For this review, take the finished solid that the model builds, in its own axes (mm). Face numbers are marked on the shaded views. A direction names the side the tool comes from. Coordinates: 2 decimals unless noted, no trailing zeros. Loops run counter-clockwise (first coordinate to the right, second up) from the corner with the lowest first, then second, coordinate; pieces in that order, holes last. Notation, with made-up numbers: (43, 47) - (62, 47) arc R20 cw to (62, 56) - close; hole circle Ø11 at (-23, 20). An arc over 180 degrees is marked (long way). One line per item, written item: value. Start each with the question number.
1. Take a section at A-A, the plane x = 4. State the section outline as (y, z) points, and give its area (3 significant figures).
2. The part is to be moulded in two halves that separate along X. For the marked faces 6, 7 and 8, say which applies: released by +X, released by -X, zero draft, split by the parting line, or undercut.
3. To check wall thickness, follow line 1 (Y direction, x = -3, z = 1.5); line 2 (Y direction, x = 1, z = 4.5); line 3 (X direction, y = -13.5, z = 3). State the ranges of each line that lie inside material, in increasing order. Write a range as from..to.
4. Insertion check: pin 1 (1.5 mm diameter, centred on y = -3, z = 1, fed in from -X); pin 2 (3 mm diameter, centred on y = 2.5, z = 2.5, fed in from +X); pin 3 (0.5 mm diameter, centred on x = 4, z = 1.5, fed in from +Y). Each pin has a flat end and moves straight along its axis. Give the tip position at first contact, or say it passes through.
5. Take a section at D-D, the plane x = -2. State the section outline as (y, z) points, and give its area (3 significant figures).
6. Take a section at B-B, the plane z = 2.5. State the section outline as (x, y) points, and give its area (3 significant figures).
7. For the marked faces 1, 2, 3, 4 and 5, list the 3-axis set-ups (+Z, -Z, +X, -X, +Y, -Y) from which the entire face can be reached by the end or side of a thin tool; tool diameter is ignored.
8. Take a section at C-C, the plane y = 16.5. State the section outline as (x, z) points, and give its area (3 significant figures).
```python
from build123d import *

# Parameters (mm, degrees)
SKETCH1_W               = 5.6
SKETCH1_H               = 40
BOSS_EXTRUDE1_DEPTH     = 4
SKETCH2_W               = 5.6
SKETCH2_H               = 2
BOSS_EXTRUDE2_DEPTH     = 4
SKETCH4_W               = 4
SKETCH4_H               = 4.2
BOSS_EXTRUDE3_DEPTH     = 1.8
MIRROR2_COPY_1_SKETCH_W = 4
MIRROR2_COPY_1_SKETCH_H = 4.2
MIRROR2_COPY_1_DEPTH    = 1.8


with BuildPart() as part:
    # Sketch1 → Boss-Extrude1 (new body)
    with BuildSketch(Plane.XY):
        Rectangle(SKETCH1_W, SKETCH1_H)
    extrude(amount=BOSS_EXTRUDE1_DEPTH)

    # Sketch2 → Boss-Extrude2 (add)
    with BuildSketch(Plane.XY.offset(4)):
        with Locations((0, -19)):
            Rectangle(SKETCH2_W, SKETCH2_H)
    extrude(amount=BOSS_EXTRUDE2_DEPTH)

    # Sketch4 → Boss-Extrude3 (add)
    with BuildSketch(Plane.ZY.offset(2.8)):
        with Locations((2, 9.6)):
            Rectangle(SKETCH4_W, SKETCH4_H)
    boss_extrude3 = extrude(amount=BOSS_EXTRUDE3_DEPTH)

    # Mirror1: Boss-Extrude3 across plane
    add(boss_extrude3.mirror(Plane.ZY))

    # Mirror2: Boss-Extrude3 across plane
    add(boss_extrude3.mirror(Plane(origin=(0, 1.1, 0), x_dir=(0, 0, 1), z_dir=(0, -1, 0))))

    # Mirror2 copy 1 sketch → Mirror2 copy 1 (add)
    with BuildSketch(Plane(origin=(2.8, 2.2, 0), x_dir=(0, 0, 1), z_dir=(1, 0, 0))):
        with Locations((2, 9.6)):
            Rectangle(MIRROR2_COPY_1_SKETCH_W, MIRROR2_COPY_1_SKETCH_H)
    extrude(amount=MIRROR2_COPY_1_DEPTH)


solid = part.part
```
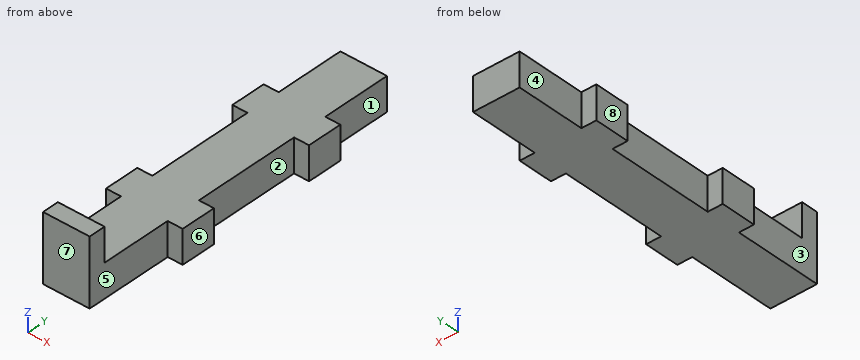
Solutions:
1. outline: (-9.5, 0) - (-5.3, 0) - (-5.3, 4) - (-9.5, 4) - close; (7.5, 0) - (11.7, 0) - (11.7, 4) - (7.5, 4) - close
1. area: 33.6 mm2
2. face 6: released by +X
2. face 7: zero draft
2. face 8: released by -X
3. line 1: -9.5..-5.3, 7.5..11.7
3. line 2: -20..-18
3. line 3: -2.8..2.8
4. pin 1: x = -2.8
4. pin 2: x = 2.8
4. pin 3: y = 11.7
5. outline: (-20, 0) - (20, 0) - (20, 4) - (-18, 4) - (-18, 8) - (-20, 8) - close
5. area: 168 mm2
6. outline: (-4.6, -9.5) - (-2.8, -9.5) - (-2.8, -20) - (2.8, -20) - (2.8, -9.5) - (4.6, -9.5) - (4.6, -5.3) - (2.8, -5.3) - (2.8, 7.5) - (4.6, 7.5) - (4.6, 11.7) - (2.8, 11.7) - (2.8, 20) - (-2.8, 20) - (-2.8, 11.7) - (-4.6, 11.7) - (-4.6, 7.5) - (-2.8, 7.5) - (-2.8, -5.3) - (-4.6, -5.3) - close
6. area: 254 mm2
7. face 1: +Z, -Z, +X, +Y
7. face 2: +Z, -Z, +X
7. face 3: +Z, -Z, -X, -Y
7. face 4: +Z, -Z, -X, +Y
7. face 5: +Z, -Z, +X, -Y
8. outline: (-2.8, 0) - (2.8, 0) - (2.8, 4) - (-2.8, 4) - close
8. area: 22.4 mm2
